Model file for the job. Use its own axes, mm. Face numbers are marked on the shaded views. A direction names the side the tool comes from. Coordinates: 2 decimals unless noted, no trailing zeros. Order: outer loops, then holes, each group sorted by start corner. A loop starts at its lowest first (then second) coordinate and runs counter-clockwise, first axis right, second up. Notation, with made-up numbers: (10, 17) - (37, 17) arc R26 cw to (37, 31) - close; hole circle Ø4 at (47, 24). An arc over 180 degrees is marked (long way). Put each result on its own line as item: value. Start each with the question number.
```python
from build123d import *

# Parameters (mm, degrees)
BOSS_EXTRUDE1_DEPTH = 10.033
BOSS_EXTRUDE2_DEPTH = 18.034
SKETCH3_R           = 16.3195
CUT_EXTRUDE1_DEPTH  = 0.762
SKETCH4_R           = 10.9982
BOSS_EXTRUDE3_DEPTH = 2.54
SKETCH5_R           = 2.54
BOSS_EXTRUDE4_DEPTH = 17.78
SKETCH6_R           = 1.27
CUT_EXTRUDE2_DEPTH  = 7.62


with BuildPart() as part:
    # Sketch1 → Boss-Extrude1 (new body)
    with BuildSketch(Plane.XY):
        Polygon((-21.082, 17.246684107), (-17.018, 21.082), (17.145, 21.082), (21.082, 17.116426271), (21.082, -17.246684107), (17.018, -21.082), (-17.145, -21.082), (-21.082, -17.116426271), align=None)
    boss_extrude1 = extrude(amount=-BOSS_EXTRUDE1_DEPTH)

    # Sketch2 → Boss-Extrude2 (add)
    with BuildSketch(Plane(origin=(0, 0, -10.033), x_dir=(-1, 0, 0), z_dir=(0, 0, -1))):
        Polygon((-21.082, 12.892006418), (-12.892006418, 21.082), (12.892006418, 21.082), (21.082, 12.892006418), (21.082, -12.892006418), (12.892006418, -21.082), (-12.892006418, -21.082), (-21.082, -12.892006418), align=None)
    extrude(amount=BOSS_EXTRUDE2_DEPTH)

    # Mirror2: Boss-Extrude1 across plane
    add(boss_extrude1.mirror(Plane.XY.offset(-18.796)))

    # Sketch3 → Cut-Extrude1 (cut)
    with BuildSketch(Plane.XY):
        Circle(SKETCH3_R)
    extrude(amount=-CUT_EXTRUDE1_DEPTH, mode=Mode.SUBTRACT)

    # Sketch4 → Boss-Extrude3 (add)
    with BuildSketch(Plane.XY.offset(-0.762)):
        Circle(SKETCH4_R)
    extrude(amount=BOSS_EXTRUDE3_DEPTH)

    # Sketch5 → Boss-Extrude4 (add)
    with BuildSketch(Plane.XY.offset(1.778)):
        Circle(SKETCH5_R)
    extrude(amount=BOSS_EXTRUDE4_DEPTH)

    # Sketch6 → Cut-Extrude2 (cut)
    with BuildSketch(Plane.XY):
        with Locations((-15.24, 15.748)):
            Circle(SKETCH6_R)
        with Locations((15.24, 15.748)):
            Circle(SKETCH6_R)
    cut_extrude2 = extrude(amount=-CUT_EXTRUDE2_DEPTH, mode=Mode.SUBTRACT)

    # Mirror3: Cut-Extrude2 across plane
    add(cut_extrude2.mirror(Plane.ZX), mode=Mode.SUBTRACT)


solid = part.part
```
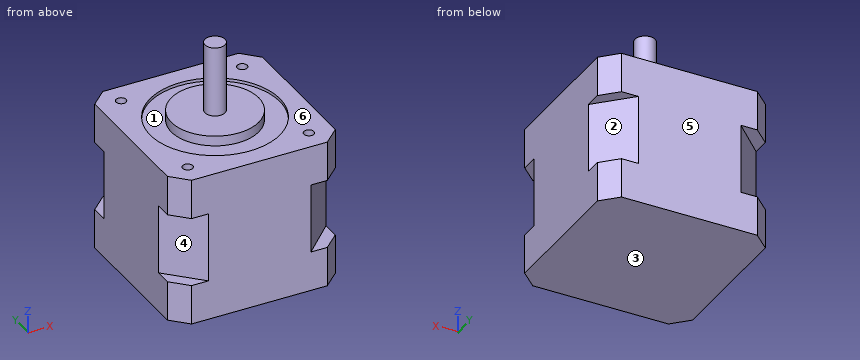
Item 1: Slice it at A-A, the plane z = -13. Give the cut face in (x, y).
Item 2: Slice it at B-B, the plane y = 0. Give the cut face in (x, z).
Item 3: Wall check: line 1 along Y through (x, z) = (0, -0.6); line 2 along Y through (x, z) = (-15.24, -1.75); line 3 along Z through (x, y) = (-18, -17.5). Give the ranges that are in metal, low to high.
Item 4: 3-axis set-ups, long thin cutter, end or side, ignore diameter. For the marked faces 5 and 6: which of +Z, -Z, +X, -X, +Y, -Y reach the whole face in a straight line?
Item 5: Pull direction Z, two halves, no side cores. Call the marked faces 1, 2, 3 and 4: pulls with the +Z half, pulls with the -Z half, needs draft (parallel to the pull), parting line crosses it, or undercut.
Item 6: Slice it at D-D, the plane z = -29. Give the cut face in (x, y) (3 decimals), plus the area to 3 significant figures.
Item 7: Flat gauge pins, fed straight in: pin 1 Ø1.5 at (y, z) = (-15, -16.5) entering from -X; pin 2 Ø4 at (x, y) = (16, 17) entering from +Z; pin 3 Ø0.8 at (x, y) = (15.5, 16) entering from +Z. Where does each tip first touch, or does it go through?
Here are the results:
1. outline: (-21.08, -12.89) - (-12.89, -21.08) - (12.89, -21.08) - (21.08, -12.89) - (21.08, 12.89) - (12.89, 21.08) - (-12.89, 21.08) - (-21.08, 12.89) - close
2. outline: (-21.08, -37.59) - (21.08, -37.59) - (21.08, 0) - (16.32, 0) - (16.32, -0.76) - (11, -0.76) - (11, 1.78) - (2.54, 1.78) - (2.54, 19.56) - (-2.54, 19.56) - (-2.54, 1.78) - (-11, 1.78) - (-11, -0.76) - (-16.32, -0.76) - (-16.32, 0) - (-21.08, 0) - close
3. line 1: y = -21.08 to -16.32, -11 to 11, 16.32 to 21.08
3. line 2: y = -21.08 to -17.02, -14.48 to 14.48, 17.02 to 21.08
3. line 3: z = -37.59 to -27.56, -10.03 to 0
4. face 5: +Z, -Z, +X, -X, +Y
4. face 6: +Z
5. face 1: pulls with the +Z half
5. face 2: undercut
5. face 3: pulls with the -Z half
5. face 4: undercut
6. outline: (-21.082, -17.116) - (-17.145, -21.082) - (17.018, -21.082) - (21.082, -17.247) - (21.082, 17.116) - (17.145, 21.082) - (-17.018, 21.082) - (-21.082, 17.247) - close
6. area: 1,750 mm^2
7. pin 1: stops at x = -19.72
7. pin 2: stops at z = 0
7. pin 3: stops at z = -7.62
